from build123d import *

# Parameters (mm, degrees)
SKETCH_1_R      = 75.00000000000001
SKETCH_1_R_2    = 60
EXTRUDE_1_DEPTH = 10
EXTRUDE_2_DEPTH = 60
EXTRUDE_START   = 55
SKETCH_3_R      = 3.0000000000000013
SKETCH_3_R_2    = 2.99999999999996
SKETCH_3_R_3    = 2.999999999999895
EXTRUDE_3_DEPTH = 5


with BuildPart() as part:
    # 草图1 → 凸台-拉伸1 (new body)
    with BuildSketch(Plane(origin=(0, 0, 0), x_dir=(1, 0, 0), z_dir=(0, 1, 0))):
        with Locations(Location((0, 0, 0), (0, 0, 270))):
            Circle(SKETCH_1_R)
        with Locations(Location((0, 0, 0), (0, 0, 270))):
            Circle(SKETCH_1_R_2, mode=Mode.SUBTRACT)
    extrude(amount=EXTRUDE_1_DEPTH)

    # 草图2 → 凸台-拉伸2 (add)
    with BuildSketch(Plane(origin=(0, 0, 0), x_dir=(1, 0, 0), z_dir=(0, 1, 0))):
        with BuildLine():
            Line((-58.09475019311125, -15), (-58.09475019311125, 15))
            Line((-58.09475019311125, 15), (-73.48469228349538, 15))
            ThreePointArc((-73.48469228349538, 15), (-75.00000000000003, 9.18e-15), (-73.48469228349538, -15))
            Line((-73.48469228349538, -15), (-58.09475019311125, -15))
        make_face()
        with BuildLine():
            Line((-14.999999999999652, -58.09475019311137), (-14.99999999999975, -73.48469228349562))
            ThreePointArc((-14.99999999999975, -73.48469228349562), (3.8762e-13, -75.00000000000017), (15.0000000000005, -73.48469228349542))
            Line((15.0000000000005, -73.48469228349542), (15.000000000000375, -58.0947501931114))
            Line((15.000000000000375, -58.0947501931114), (-14.999999999999652, -58.09475019311137))
        make_face()
        with BuildLine():
            Line((58.094750193111345, -14.999999999999556), (58.09475019311114, 15.000000000000444))
            Line((58.09475019311114, 15.000000000000444), (73.48469228349526, 15.000000000000444))
            ThreePointArc((73.48469228349526, 15.000000000000444), (75.00000000000001, 4.5589e-13), (73.48469228349548, -14.999999999999556))
            Line((73.48469228349548, -14.999999999999556), (58.094750193111345, -14.999999999999556))
        make_face()
        with BuildLine():
            Line((-14.999999999999833, 58.09475019311096), (-14.999999999999943, 73.4846922834952))
            ThreePointArc((-14.999999999999943, 73.4846922834952), (2.7105e-13, 75.00000000000016), (15.000000000000528, 73.48469228349539))
            Line((15.000000000000528, 73.48469228349539), (15.00000000000043, 58.09475019311115))
            Line((15.00000000000043, 58.09475019311115), (-14.999999999999833, 58.09475019311096))
        make_face()
    extrude(amount=EXTRUDE_2_DEPTH)

    # 草图3 → 凸台-拉伸3 (add)
    # profile 1 of 4: a face of its own
    with BuildSketch(Plane(origin=(0, 0, 0), x_dir=(1, 0, 0), z_dir=(0, 1, 0)).offset(EXTRUDE_START)):
        with BuildLine():
            Line((73.48469228349529, 15.000000000000448), (58.09475019311114, 15.000000000000444))
            Line((58.09475019311114, 15.000000000000444), (40, 15.000000000000014))
            ThreePointArc((40, 15.000000000000014), (25, 1.653e-14), (40, -14.999999999999986))
            Line((40, -14.999999999999986), (58.094750193111345, -14.999999999999556))
            Line((58.094750193111345, -14.999999999999556), (73.48469228349545, -14.999999999999556))
            ThreePointArc((73.48469228349545, -14.999999999999556), (75.00000000000001, 4.5172e-13), (73.48469228349529, 15.000000000000448))
        make_face()
        with Locations(Location((40, 1.47e-14, 0), (0, 0, 270))):
            Circle(SKETCH_3_R, mode=Mode.SUBTRACT)
    # profile 2 of 4: a face of its own
    with BuildSketch(Plane(origin=(0, 0, 0), x_dir=(1, 0, 0), z_dir=(0, 1, 0)).offset(EXTRUDE_START)):
        with BuildLine():
            Line((-73.48469228349538, -14.999999999999998), (-58.09475019311125, -15))
            Line((-58.09475019311125, -15), (-40, -15))
            ThreePointArc((-40, -15), (-25, 0), (-40, 15))
            Line((-40, 15), (-58.09475019311125, 15))
            Line((-58.09475019311125, 15), (-73.48469228349538, 15))
            ThreePointArc((-73.48469228349538, 15), (-75.00000000000003, 9.18e-15), (-73.48469228349538, -14.999999999999998))
        make_face()
        with Locations(Location((-40, 0, 0), (0, 0, 270))):
            Circle(SKETCH_3_R, mode=Mode.SUBTRACT)
    # profile 3 of 4: a face of its own
    with BuildSketch(Plane(origin=(0, 0, 0), x_dir=(1, 0, 0), z_dir=(0, 1, 0)).offset(EXTRUDE_START)):
        with BuildLine():
            Line((-14.999999999999833, 58.09475019311096), (-14.99999999999975, 73.4846922834952))
            ThreePointArc((-14.99999999999975, 73.4846922834952), (3.7097e-13, 74.99999999999982), (15.000000000000554, 73.48469228349539))
            Line((15.000000000000554, 73.48469228349539), (15.00000000000043, 58.09475019311115))
            Line((15.00000000000043, 58.09475019311115), (14.999999999999867, 39.99999999999992))
            ThreePointArc((14.999999999999867, 39.99999999999992), (6.281e-14, 25.00000000000015), (-15.00000000000016, 39.99999999999973))
            Line((-15.00000000000016, 39.99999999999973), (-14.999999999999833, 58.09475019311096))
        make_face()
        with Locations(Location((-3.469e-14, 40.00000000000005, 0), (0, 0, 270))):
            Circle(SKETCH_3_R_2, mode=Mode.SUBTRACT)
    # profile 4 of 4: a face of its own
    with BuildSketch(Plane(origin=(0, 0, 0), x_dir=(1, 0, 0), z_dir=(0, 1, 0)).offset(EXTRUDE_START)):
        with BuildLine():
            Line((-14.999999999999652, -58.09475019311137), (-14.999999999999867, -40.000000000000135))
            ThreePointArc((-14.999999999999867, -40.000000000000135), (2.6731e-13, -24.99999999999991), (15.00000000000016, -40.00000000000016))
            Line((15.00000000000016, -40.00000000000016), (15.000000000000375, -58.0947501931114))
            Line((15.000000000000375, -58.0947501931114), (15.0000000000005, -73.48469228349542))
            ThreePointArc((15.0000000000005, -73.48469228349542), (3.8762e-13, -75.00000000000017), (-14.99999999999975, -73.48469228349562))
            Line((-14.99999999999975, -73.48469228349562), (-14.999999999999652, -58.09475019311137))
        make_face()
        with Locations(Location((2.5674e-13, -40.000000000000036, 0), (0, 0, 270))):
            Circle(SKETCH_3_R_3, mode=Mode.SUBTRACT)
    extrude(amount=EXTRUDE_3_DEPTH)


solid = part.part
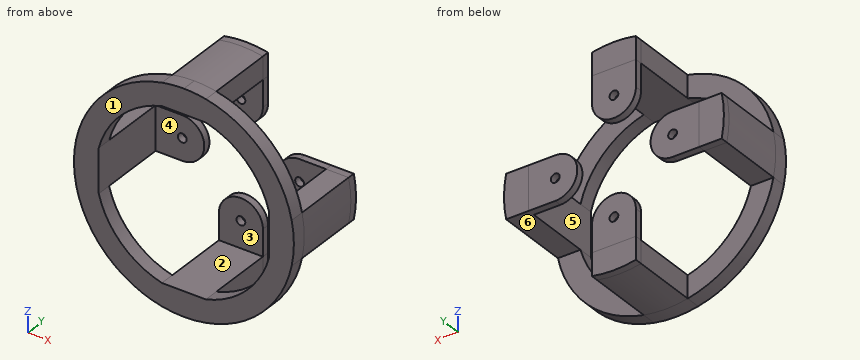
Here's how the part is built. I have some questions about the finished solid (model axes, mm). Face numbers are marked on the shaded views. A direction names the side the tool comes from. Round coordinates to 2 decimals unless told otherwise and drop trailing zeros. Loops run counter-clockwise (first coordinate to the right, second up) from the corner with the lowest first, then second, coordinate; pieces in that order, holes last. Notation, with made-up numbers: M 73,75.5 L 100,75.5 A14 ccw 100,85.5 Z; hole C -16.5,-17.5 d1. An arc over 180 degrees is marked long. Write each question's results on one line, items separated by ' | '. Start each with the question number.
(1) I want a section at B-B (z = 0). Please give me the cut outline in (x, y), then the cut area to 3 significant figures.
(2) On a 3-axis mill with a long thin cutter (end or side, diameter ignored), from which of +Z, -Z, +X, -X, +Y, -Y can I reach the whole of each face in a straight line? I mean the marked faces 3, 4, 5 and 6. Say none if no direction works.
(3) I want a section at D-D (x = -63). Please give me the cut outline in (y, z).
(4) Will these pins go through, and if not, where does the flat tip stop? P1, Ø9, axis at x = -46.5, z = -4, coming from the -Y side; P2, Ø5, axis at x = 19.5, z = 58, coming from the +Y side; P3, Ø6, axis at y = 39.5, z = 53, coming from the -X side; P4, Ø4, axis at y = 58.5, z = 64, coming from the +X side.
(5) If I drill on probe 1 along X at (y, z) = (57.4, 0); probe 2 along Y at (x, z) = (43, 55); probe 3 along X at (y, z) = (26.5, -66), over which ranges is the centre line in solid material (lowest first)? Write a range as from..to.
(6) Thinking about a two-plate mould opening in X: for the marked faces 1 and 2, which applies, pulls with the +X half, pulls with the -X half, needs draft (parallel to the pull), parting line crosses it, or undercut?
(7) I want a section at C-C (z = 19.5). Please give me the cut outline in (x, y).
(8) I want a section at A-A (y = 28). Please give me the cut outline in (x, z), then the cut area to 3 significant figures.
Solved:
1) outline: M -75,0 L -58.09,0 L -58.09,55 L -43,55 L -43,60 L -75,60 Z; M -37,55 L -25,55 L -25,60 L -37,60 Z; M 25,55 L 37,55 L 37,60 L 25,60 Z; M 43,55 L 58.09,55 L 58.09,0 L 75,0 L 75,60 L 43,60 Z | area: 2,300 mm²
2) face 3: +X, -X, -Y | face 4: +Z, -Z, -Y | face 5: -Y | face 6: -Z, +X, -X, +Y
3) outline: M 0,-40.69 L 10,-40.69 L 10,-15 L 60,-15 L 60,15 L 10,15 L 10,40.69 L 0,40.69 Z
4) P1: stops at y = 55 | P2: stops at y = 10 | P3: passes through | P4: stops at x = 15
5) probe 1: x = -75..-43, -37..-25, 25..37, 43..75 | probe 2: y = 0..10 | probe 3: x = -15..15
6) face 1: needs draft | face 2: undercut
7) outline: M -72.42,0 L -56.74,0 L -56.74,10 L -72.42,10 Z; M 56.74,0 L 72.42,0 L 72.42,10 L 56.74,10 Z
8) outline: M -73.48,-15 L -58.09,-15 L -58.09,15 L -73.48,15 A75 ccw Z; M -15,-73.48 A75 ccw 15,-73.48 L 15,-58.09 L -15,-58.09 Z; M -15,58.09 L 15,58.09 L 15,73.48 A75 ccw -15,73.48 Z; M 58.09,-15 L 73.48,-15 A75 ccw 73.48,15 L 58.09,15 Z | area: 1,970 mm²
